```python
from build123d import *

# Parameters (mm, degrees)
F1_DEPTH = 8
F3_DEPTH = 10
F5_DEPTH = 10
F6_W     = 2
F6_H     = 4
F7_DEPTH = 2


with BuildPart() as f1:
    # F0 (on Front) → F1 (new body)
    with BuildSketch(Plane.XZ):
        Polygon((10, 14), (-10, 14), (-10, 13.9871324164), align=None)
        with BuildLine():
            Line((-10, 13.9871324164), (-10, 14))
            add(Edge.make_bspline(
                [(-10, 14), (-10.0013069916, 13.9957099885), (-10.0026139149, 13.9914199529), (-10.0039207687, 13.9871298939)],
                knots=[0, 0, 0, 0, 0.0005634153, 0.0005634153, 0.0005634153, 0.0005634153], degree=3))
            Line((-10.0039207687, 13.9871298939), (-10, 13.9871324164))
        make_face()
        with BuildLine():
            add(Edge.make_bspline(
                [(-10, 14), (-10.0013069916, 13.9957099885), (-10.0026139149, 13.9914199529), (-10.0039207687, 13.9871298939)],
                knots=[0, 0, 0, 0, 0.0005634153, 0.0005634153, 0.0005634153, 0.0005634153], degree=3))
            Line((-10, 14), (-18.0412381887, 13.9819588512))
            Line((-18.0412381887, 13.9819588512), (-10.0039207687, 13.9871298939))
        make_face()
        with BuildLine():
            add(Edge.make_bspline(
                [(16.5979396552, 25.1705870032), (16.4242079195, 21.7814034546), (16.1292929338, 16.0281597324), (17.954552315, 8.034475712), (12.8387475955, 11.8710784645), (10, 14)],
                knots=[0, 0, 0, 0, 0.3895409215, 0.6612577422, 1, 1, 1, 1], degree=3))
            Line((10, 14), (10, 6.6676748447))
            add(Edge.make_bspline(
                [(10, 6.6676748447), (10.2523378817, 5.6781345951), (12.0047533576, 2.0571975496), (22.7187939676, 0.2071940627), (26.2944872886, 12.0093761919), (24.7818586393, 20.5559387988), (24.5979396552, 25.1705870032)],
                knots=[0.1642768485, 0.1642768485, 0.1642768485, 0.1642768485, 0.2408562316, 0.4776886549, 0.7182430468, 1, 1, 1, 1], degree=3))
            Line((24.5979396552, 25.1705870032), (16.5979396552, 25.1705870032))
        make_face()
        with BuildLine():
            Line((10, 6.6676748447), (10, 14))
            add(Edge.make_bspline(
                [(10, 14), (9.7266030818, 11.3954202783), (9.4586888759, 8.790420511), (10, 6.6676748447)],
                knots=[0, 0, 0, 0, 0.1642768485, 0.1642768485, 0.1642768485, 0.1642768485], degree=3))
        make_face()
        with BuildLine():
            add(Edge.make_bspline(
                [(10, 14), (9.7266030818, 11.3954202783), (9.4586888759, 8.790420511), (10, 6.6676748447)],
                knots=[0, 0, 0, 0, 0.1642768485, 0.1642768485, 0.1642768485, 0.1642768485], degree=3))
            Line((10, 14), (-10, 13.9871324164))
            Line((-10, 13.9871324164), (-10, -14))
            Line((-10, -14), (10, -14))
            Line((10, -14), (10, 6.6676748447))
        make_face()
        with BuildLine():
            add(Edge.make_bspline(
                [(-10.0039207687, 13.9871298939), (-10.557530177, 12.1697751658), (-11.6304994418, 8.5580895587), (-12.7269597722, 3.2080619518), (-15.9483733573, -2.8154175848), (-17.9189211947, -6.9664320189), (-18.3122973873, -9.2296893574)],
                knots=[0.0005634153, 0.0005634153, 0.0005634153, 0.0005634153, 0.2392373891, 0.4737911443, 0.7359345398, 1, 1, 1, 1], degree=3))
            Line((-10.0039207687, 13.9871298939), (-18.0412381887, 13.9819588512))
            add(Edge.make_bspline(
                [(-25.9793829173, -6.9458768703), (-25.2539642188, -4.5676118012), (-23.8093664017, 0.1684620471), (-19.5153648693, 6.2164021065), (-18.5387466084, 11.3611326258), (-18.0412381887, 13.9819588512)],
                knots=[0, 0, 0, 0, 0.3310306201, 0.65921393, 1, 1, 1, 1], degree=3))
            Line((-25.9793829173, -6.9458768703), (-18.3122973873, -9.2296893574))
        make_face()
    extrude(amount=F1_DEPTH)

    # F2 (on face) → F3 (join)
    with BuildSketch(Plane(origin=(-10, 0, 0), x_dir=(0, -1, 0), z_dir=(-1, 0, 0))):
        with BuildLine():
            Line((8, -14), (0, -14))
            add(Edge.make_bspline(
                [(0, -14), (0.2045836759, -15.6157837158), (0.6192637374, -18.8902476344), (-2.6809411284, -22.8970011823), (-4.6665400492, -28.7619394429), (-5.2928585425, -32.41202967), (-5.5954085566, -34.1871318147)],
                knots=[0, 0, 0, 0, 0.2346269916, 0.4754883695, 0.745007012, 1, 1, 1, 1], degree=3))
            Line((-5.5954085566, -34.1871318147), (0, -36.3530965155))
            add(Edge.make_bspline(
                [(8, -14), (8.1062479665, -15.4020488735), (8.3373620016, -18.4518314863), (6.2753772925, -24.1836933573), (1.2807636539, -30.1416891817), (0.4114158447, -34.3578251248), (0, -36.3530965155)],
                knots=[0, 0, 0, 0, 0.2121639716, 0.4615060148, 0.7451596188, 1, 1, 1, 1], degree=3))
        make_face()
    extrude(amount=-F3_DEPTH)

    # F4 (on face) → F5 (join)
    with BuildSketch(Plane.YZ):
        with BuildLine():
            add(Edge.make_bspline(
                [(0, -14), (-0.8240515576, -15.4606959655), (-2.3272345442, -18.1252934548), (-4.0109662696, -20.975339063), (-4.9011507822, -25.8671770363), (-4.9008100664, -31.9777881879), (-5.3812911094, -34.640359184), (-5.592783913, -35.811856389)],
                knots=[0, 0, 0, 0, 0.2049146304, 0.3738081441, 0.5819768139, 0.8160801398, 1, 1, 1, 1], degree=3))
            Line((0, -14), (-8, -14))
            add(Edge.make_bspline(
                [(-8, -14), (-8.789860184, -15.0975567751), (-10.5069200527, -17.4835115686), (-11.2071319942, -23.284631647), (-12.8483158405, -28.5406582263), (-12.3418277002, -32.3002507673), (-12.0876291767, -34.1871318147)],
                knots=[0, 0, 0, 0, 0.2229102117, 0.4845796593, 0.741318544, 1, 1, 1, 1], degree=3))
            Line((-12.0876291767, -34.1871318147), (-5.592783913, -35.811856389))
        make_face()
    extrude(amount=F5_DEPTH)

    # F6 (on face) → F7 (join)
    with BuildSketch(Plane(origin=(0, 0, 0), x_dir=(-1, 0, 0), z_dir=(0, 1, 0))):
        with Locations((-17.5979396552, 27.1705870032)):
            Rectangle(F6_W, F6_H)
    extrude(amount=-F7_DEPTH)


solid = f1.part
```
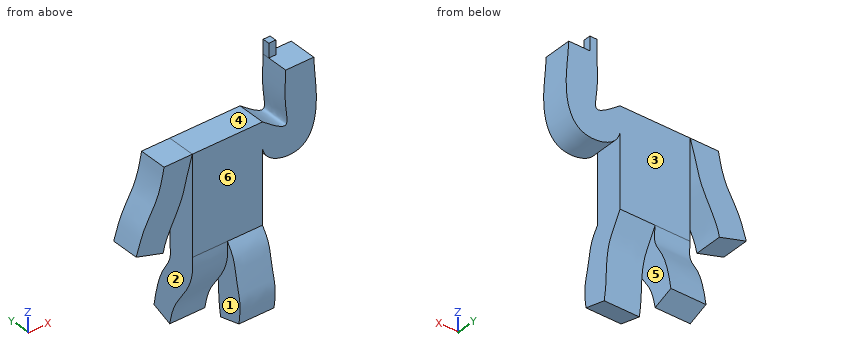
The model under review builds one solid part; all positions refer to its coordinate system, in mm. Face numbers are marked on the shaded views. A direction names the side the tool comes from. Round coordinates to 2 decimals unless told otherwise and drop trailing zeros. Answer as CSV lines item,"result". Start each with the question number.
(1) For the marked faces 4, 5 and 6, list the 3-axis set-ups (+Z, -Z, +X, -X, +Y, -Y) from which the entire face can be reached by the end or side of a thin tool; tool diameter is ignored.
(2) For pin 1 Ø3.5 at (y, z) = (-6, -11) entering from +X; pin 2 Ø2 at (y, z) = (-1.5, 28) entering from -X; pin 3 Ø3 at (y, z) = (1, -25) entering from +X; pin 4 Ø1 at (x, z) = (0, 15) entering from -Y, all flat-tipped, find the tip position at first contact; note any pin that passes through.
(3) Draft analysis for pull direction X (two halves, no side actions). For the marked faces 1, 2 and 3, state which applies: pulls with the +X half, pulls with the -X half, needs draft (parallel to the pull), parting line crosses it, or undercut.
(4) To check wall thickness, follow line 1 (X direction, y = -7.5, z = -33); line 2 (X direction, y = -3.5, z = 11.5); line 3 (Y direction, x = -6.5, z = -10). State the ranges of each line that lie inside material, in increasing order.
Worked answers:
1,face 4,"+Z, -X, +Y, -Y"
1,face 5,"-Z, +X, +Y"
1,face 6,"+Z, +X, -X, -Y"
2,pin 1,"x = 10"
2,pin 2,"x = 16.6"
2,pin 3,"x = 0"
2,pin 4,"through"
3,face 1,"pulls with the -X half"
3,face 2,"undercut"
3,face 3,"needs draft"
4,line 1,"0 to 10"
4,line 2,"-18.53 to -10.75, -10 to 13.46, 16.99 to 25.26"
4,line 3,"-8 to 0"
